Geometry check sheet. Reference: the model listing, model coordinates, mm. Give positions to 0.01 mm unless a question says otherwise; leave off trailing zeros. Write each loop counter-clockwise with the first axis right and the second up, starting at its lowest first coordinate (ties: lowest second). Pieces come first, ordered by that corner, then holes. Notation, with made-up numbers: (30.25, 62) - (35.25, 62) arc R18 cw to (35.25, 96) - close; hole circle Ø5 at (32.5, -31.75). An arc over 180 degrees is marked (long way). One line per question, with ' | ' between items. Start each with the question number.
Q1. Section check A-A on x = 1.5. Record the boundary of the cut face in (y, z), and give its area (3 significant figures).
Q2. Thickness scan on L1, parallel to X at y = -34, z = 0.2; L2, parallel to Y at x = 2.5, z = 1.25; L3, parallel to Y at x = -2.25, z = 1.5. Record the ranges inside material, lowest first. Write a range as [from, to].
Q3. Section check B-B on y = -26. Record the boundary of the cut face in (x, z).
Q4. Gauge pin test, flat ends, axial feed: P1, Ø1.3, axis at y = -52, z = 2, coming from the -X side; P2, Ø1, axis at x = -2, y = -10.5, coming from the -Z side; P3, Ø1.5, axis at y = -46.5, z = 1, coming from the +X side; P4, Ø0.7, axis at x = -3, z = 1.5, coming from the -Y side. Record the tip position at first contact, or that the pin passes through.
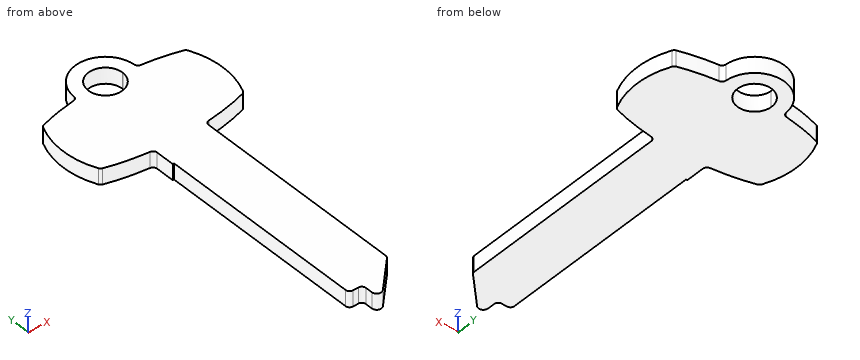
```python
from build123d import *

# Parameters (mm, degrees)
F1_DEPTH = 2.54
F3_DEPTH = 2.54
F4_R     = 0.635


with BuildPart() as f1:
    # F0 (on Top) → F1 (new body)
    with BuildSketch(Plane.XY):
        with BuildLine():
            ThreePointArc((2.7292355161, -0.0830887952), (0, -2.7305), (-2.7292355161, -0.0830887952))
            add(Edge.make_bspline(
                [(-2.7292355161, -0.0830887952), (-3.7940557667, -0.1483067369), (-4.8315057716, -0.2637606285)],
                knots=[1.7238043068, 1.7238043068, 1.7238043068, 1.8439930848, 1.8439930848, 1.8439930848], degree=2, weights=[1, 0.9981948755, 1]))
            add(Edge.make_bspline(
                [(-4.8315057716, -0.2637606285), (-8.5391367, -0.6763688673), (-11.4920446345, -1.6577838797)],
                knots=[1.8439930848, 1.8439930848, 1.8439930848, 2.2675908503, 2.2675908503, 2.2675908503], degree=2, weights=[1, 0.9776543376, 1]))
            ThreePointArc((-11.4920446345, -1.6577838797), (-12.7508, -7.112), (-11.4920446345, -12.5662161203))
            add(Edge.make_bspline(
                [(-11.4920446345, -12.5662161203), (0, -16.3856596579), (11.4920446345, -12.5662161203)],
                knots=[4.0155944569, 4.0155944569, 4.0155944569, 5.4091835039, 5.4091835039, 5.4091835039], degree=2, weights=[1, 0.766903279, 1]))
            ThreePointArc((11.4920446345, -12.5662161203), (12.7508, -7.112), (11.4920446345, -1.6577838797))
            add(Edge.make_bspline(
                [(11.4920446345, -1.6577838797), (8.5391367, -0.6763688673), (4.8315057716, -0.2637606285)],
                knots=[0.8740018033, 0.8740018033, 0.8740018033, 1.2975995688, 1.2975995688, 1.2975995688], degree=2, weights=[1, 0.9776543376, 1]))
            add(Edge.make_bspline(
                [(4.8315057716, -0.2637606285), (3.7940557667, -0.1483067369), (2.7292355161, -0.0830887952)],
                knots=[1.2975995688, 1.2975995688, 1.2975995688, 1.4177883468, 1.4177883468, 1.4177883468], degree=2, weights=[1, 0.9981948755, 1]))
        make_face()
        with BuildLine():
            ThreePointArc((-2.7292355161, -0.0830887952), (-0.0415492082, 2.7301838607), (2.7305, 0))
            ThreePointArc((2.7305, 0), (2.7301838607, -0.0415492082), (2.7292355161, -0.0830887952))
            add(Edge.make_bspline(
                [(4.8315057716, -0.2637606285), (3.7940557667, -0.1483067369), (2.7292355161, -0.0830887952)],
                knots=[1.2975995688, 1.2975995688, 1.2975995688, 1.4177883468, 1.4177883468, 1.4177883468], degree=2, weights=[1, 0.9981948755, 1]))
            ThreePointArc((4.8315057716, -0.2637606285), (0, 4.8387), (-4.8315057716, -0.2637606285))
            add(Edge.make_bspline(
                [(-2.7292355161, -0.0830887952), (-3.7940557667, -0.1483067369), (-4.8315057716, -0.2637606285)],
                knots=[1.7238043068, 1.7238043068, 1.7238043068, 1.8439930848, 1.8439930848, 1.8439930848], degree=2, weights=[1, 0.9981948755, 1]))
        make_face()
    extrude(amount=F1_DEPTH)

    # F2 (on Top) → F3 (join, through all)
    with BuildSketch(Plane.XY):
        with BuildLine():
            add(Edge.make_bspline(
                [(-4.1402, -14.0312996195), (0, -14.4220670272), (4.1402, -14.0312996195)],
                knots=[4.4790722282, 4.4790722282, 4.4790722282, 4.9457057325, 4.9457057325, 4.9457057325], degree=2, weights=[1, 0.9729048959, 1]))
            Line((-4.1402, -14.0312996195), (-4.1402, -17.5872996195))
            Line((-4.1402, -17.5872996195), (-3.937, -17.5872996195))
            Line((-3.937, -17.5872996195), (-3.937, -50.6072996195))
            Line((-3.937, -50.6072996195), (-1.778, -50.6072996195))
            Line((-1.778, -50.6072996195), (-1.778, -52.3998688849))
            ThreePointArc((-1.778, -52.3998688849), (-1.3076047755, -53.1038650887), (-0.4771846327, -52.9386842522))
            Line((-0.4771846327, -52.9386842522), (3.9170153673, -48.5444842522))
            ThreePointArc((3.9170153673, -48.5444842522), (4.0821962038, -48.2972736604), (4.1402, -48.0056688849))
            Line((4.1402, -48.0056688849), (4.1402, -14.0312996195))
        make_face()
    extrude(amount=F3_DEPTH)

    # F4
    f4_edges = [f1.edges().sort_by_distance(p)[0] for p in [
        (-4.1402, -14.0313, 1.27),
        (4.1402, -14.0313, 1.27),
        (11.492045, -12.566216, 1.27),
        (11.492045, -1.657784, 1.27),
        (-11.492045, -1.657784, 1.27),
        (-11.492045, -12.566216, 1.27),
        (-3.937, -50.6073, 1.27),
        (-1.778, -50.6073, 1.27),
        (4.831506, -0.263761, 1.27),
        (-4.831506, -0.263761, 1.27),
    ]]
    fillet(f4_edges, radius=F4_R)


solid = f1.part
```
Working result:
1) outline: (-50.96, 0) - (-2.28, 0) - (-2.28, 2.54) - (-50.96, 2.54) - close; (2.28, 0) - (4.6, 0) - (4.6, 2.54) - (2.28, 2.54) - close | area: 130 mm2
2) L1: x = [-3.94, 4.14] | L2: y = [-49.96, -1.1], [1.1, 4.14] | L3: y = [-50.63, -1.55], [1.55, 4.28]
3) outline: (-3.94, 0) - (4.14, 0) - (4.14, 2.54) - (-3.94, 2.54) - close
4) P1: stops at x = -1.78 | P2: stops at z = 0 | P3: stops at x = 4.14 | P4: stops at y = -50.61
